Geometry: final body of the model. Coordinates: model frame, mm. A direction names the side the tool comes from. Round coordinates to 2 decimals unless told otherwise and drop trailing zeros. Write each loop counter-clockwise with the first axis right and the second up, starting at its lowest first coordinate (ties: lowest second). Pieces come first, ordered by that corner, then holes. Notation, with made-up numbers: (28.25, -11) -> (68.25, -11) arc R20 ccw to (68.25, 26) -> close; hole circle Ø3 at (-15.5, 40.25). An arc over 180 degrees is marked (long way). Use one line per item in the form item = value. Start each with the question number.
1. Line query: L1, parallel to Z at x = 7.75, y = -2.5; L2, parallel to Z at x = -8.5, y = 26. Output: solid intervals per line, ascending.
2. Draft query along Z for faces 1 (the face through (10, -36, 0)), 2 (the face through (0, -37, -9.25)), 3 (the face through (0, -36, -10)), 4 (the face through (-9.583, 34.043, -0.787)). Return one class per face: pulls with the +Z half, pulls with the -Z half, needs draft (parallel to the pull), parting line crosses it, or undercut.
3. Cut plane D-D, the plane y = 32.5. Return the cut outline in (x, z), plus the area to 3 significant figures.
4. Cut plane A-A, the plane x = 3.25. Return the cut outline in (y, z), plus the area to 3 significant figures.
5. Pin query (flat end, axial travel): pin 1 Ø4 at (x, z) = (5.5, 1) entering from +Y. Return the tip coordinate at first contact, or that it passes through.
6. Reachability of faces 5 (the face through (-10, -36, 0)), 6 (the face through (9.25, -37, 0)) from +Z, -Z, +X, -X, +Y, -Y: full face, straight path, thin tool, end or side. Return the list, or none.
7. Cut plane B-B, the plane z = -7. Return the cut outline in (x, y), plus the area to 3 significant figures.
8. Cut plane C-C, the plane y = 13. Return the cut outline in (x, z), plus the area to 4 significant figures.
Autodesk Inventor part; units mm, degrees
ref_plane "YZ Plane" through (0, 0, 0) normal (1, 0, 0) x (0, 1, 0)
ref_plane "XZ Plane" through (0, 0, 0) normal (0, 1, 0) x (-1, 0, 0)
ref_plane "XY Plane" through (0, 0, 0) normal (0, 0, 1) x (1, 0, 0)
sketch "Эскиз1" plane through (0, 0, 0) normal (0, 1, 0) x (-1, 0, 0)
  line L0 (-10, -10) -> (10, -10)
  line L1 (10, -10) -> (10, 10)
  line L2 (10, 10) -> (-10, 10)
  line L3 (-10, 10) -> (-10, -10)
  line L4 (-10, -10) -> (10, 10) construction
  line L5 (10, -10) -> (-10, 10) construction
  line L6 (-9.25, -9.25) -> (9.25, -9.25)
  line L7 (9.25, -9.25) -> (9.25, 9.25)
  line L8 (9.25, 9.25) -> (-9.25, 9.25)
  line L9 (-9.25, 9.25) -> (-9.25, -9.25)
  line L10 (-9.25, -9.25) -> (9.25, 9.25) construction
  line L11 (9.25, -9.25) -> (-9.25, 9.25) construction
  point P0 (0, 0)
  dimension "d0" = 20
  dimension "d1" = 20
  dimension "d2" = 18.5
  dimension "d3" = 18.5
extrude "Выдавливание1" add sketch "Эскиз1" along normal blind 50 and the other way blind 120
sketch "Эскиз2" plane through (10, -120, 10) normal (1, 0, 0) x (0, 0, -1)
  line L0 (20, 0) -> (20, 170)
  line L1 (20, 170) -> (0, 135.359)
  line L2 (0, 0) -> (0, 170)
  line L3 (20, 170) -> (60, 170) construction
  line L4 (20, 170) -> (0, 170)
  line L5 (0, 135.359) -> (0, 170)
  line L6 (0, 170) -> (20, 170)
  point P0 (10, 120)
  dimension "d6" = 120
extrude "Выдавливание2" cut sketch "Эскиз2" against normal blind 50
Outcome:
q1.L1 = -10 to -9.25, 9.25 to 10
q1.L2 = -10 to -9.25
q2.face_1 = needs draft
q2.face_2 = undercut
q2.face_3 = pulls with the -Z half
q2.face_4 = pulls with the +Z half
q3.outline = (-10, -10) -> (10, -10) -> (10, 0.1) -> (9.25, 0.1) -> (9.25, -9.25) -> (-9.25, -9.25) -> (-9.25, 0.1) -> (-10, 0.1) -> close
q3.area = 29.0 mm^2
q4.outline = (-120, -10) -> (50, -10) -> (48.7, -9.25) -> (-120, -9.25) -> close; (-120, 9.25) -> (16.66, 9.25) -> (15.36, 10) -> (-120, 10) -> close
q4.area = 229 mm^2
q5.pin_1 = through
q6.face_5 = +Z, -Z, -X, +Y, -Y
q6.face_6 = +Y, -Y
q7.outline = (-10, -120) -> (-9.25, -120) -> (-9.25, 44.8) -> (-10, 44.8) -> close; (9.25, -120) -> (10, -120) -> (10, 44.8) -> (9.25, 44.8) -> close
q7.area = 247 mm^2
q8.outline = (-10, -10) -> (10, -10) -> (10, 10) -> (-10, 10) -> close; hole (-9.25, -9.25) -> (9.25, -9.25) -> (9.25, 9.25) -> (-9.25, 9.25) -> close
q8.area = 57.75 mm^2
